Geometry check sheet. Reference: the model listing, model coordinates, mm. Face numbers are marked on the shaded views. A direction names the side the tool comes from. Coordinates: 2 decimals unless noted, no trailing zeros. Write each loop counter-clockwise with the first axis right and the second up, starting at its lowest first coordinate (ties: lowest second). Pieces come first, ordered by that corner, then holes. Notation, with made-up numbers: (62, 45) -> (90, 45) arc R19 cw to (90, 74) -> close; hole circle Ø5 at (37, 17). An arc over 180 degrees is marked (long way). Use a Markdown table: item, result.
Autodesk Inventor part; units mm, degrees
ref_plane "Work Plane1" through (29, 0, 0) normal (0, -1, 0) x (1, 0, 0)
ref_plane "YZ Plane" through (0, 0, 0) normal (1, 0, 0) x (0, 1, 0)
ref_plane "XZ Plane" through (0, 0, 0) normal (0, 1, 0) x (-1, 0, 0)
sketch "Sketch1" plane through (0, 0, 0) normal (0, 0, 1) x (1, 0, 0)
  line L0 (0.1133, 0) -> (20, 0)
  line L1 (20, 0) -> (20, 3)
  line L2 (20, 3) -> (3, 3)
  line L3 (3, 3) -> (2.3864, 3)
  line L4 (2.3864, 3) -> (0, 3)
  line L5 (0, 3) -> (0, 5.25)
  line L6 (0, 5.25) -> (-3.3, 5.25)
  line L7 (-3.3, 5.25) -> (-3.3, 2.3094)
  line L8 (-3.3, 2.3094) -> (-1.22, 2.3094)
  line L9 (-1.22, 2.3094) -> (0.1133, 0)
  line L10 (-7.96, 0) -> (24.66, 0)
  line L11 (0, -1.05) -> (0, 6.3)
  line L12 (3, 3) -> (0, 3) construction
  dimension "d1" = 17
  dimension "d2" = 0.6136
  dimension "d3" = 3.3
  dimension "d4" = 2.08
  dimension "d5" = 60
  dimension "d6" = 6
  dimension "d7" = 6
  dimension "d8" = 4.6188
  dimension "d9" = 10.5
  dimension "d26" = 20
revolve "Body" add sketch "Sketch1" angle 360 about axis through (0.1133, 0, 0) along (1, 0, 0) contours L9 L11 L4 L3 L2 L1 L0 | L9 L8 L7 L6 L5 L11
sketch "Sketch2" plane through (-3.3, 0, 0) normal (-1, 0, 0) x (0, 0, 1)
  circle A0 centre (0, 0) radius 2.3094
  line L0 (0, -7.35) -> (0, 7.35)
  line L1 (-7.35, 0) -> (7.35, 0)
  line L2 (2.3094, 0) -> (1.1547, -2)
  line L3 (1.1547, -2) -> (-1.1547, -2)
  line L4 (-1.1547, -2) -> (-2.3094, 0)
  line L5 (-2.3094, 0) -> (-1.1547, 2)
  line L6 (-1.1547, 2) -> (1.1547, 2)
  line L7 (1.1547, 2) -> (2.3094, 0)
extrude "Slot" add sketch "Sketch2" against normal up to next contours L7 A0 | A0 L2 | L6 L0 A0 | A0 L0 L3 | L0 L6 A0 | A0 L3 L0 | L4 A0 | A0 L5
fillet "Fillet1" radius 2.56 1 edges at (-3.3, -5.25, 0)
thread "Thread"
chamfer "Chamfer1" distance 0.6135 distance2 0.6135 1 edges at (20, -3, 0) measured on face at (20, 1.0659, 1.0214)
ref_plane "Work Plane1" through (29, 0, 0) normal (0, -1, 0) x (1, 0, 0)
fillet "Fillet2" radius 0.5 1 edges at (0, -3, 0)
equation "\"d1\" = GEL"
equation "\"d3\" = KOH"
equation "\"d4\" = INTI"
equation "\"d6\" = GD"
equation "\"d7\" = BDM"
equation "\"d8\" = 1.1547 * SW"
equation "\"d9\" = KOD"
equation "\"d26\" = NLG"
equation "\"d30\" = R"
equation "\"d17\" = RR"
equation "\"d13\" = GEL"
equation "\"d15\" = -0.5 * SPD + 0.5 * GD"
equation "\"d16\" = GUL"
equation "\"GD\" = NND"
equation "\"NLG\" = 20"
equation "\"GEL\" = 17"
equation "\"KOD\" = 10.5"
equation "\"KOH\" = 3.3"
equation "\"INTI\" = 2.08"
equation "\"GAL\" = 0.61345 * PTC"
equation "\"GUL\" = 0.61345 * PTC"
equation "\"BDM\" = NND"
equation "\"SW\" = 4"
equation "\"RR\" = 2.56"
equation "\"SPD\" = NND - 1.2269 * PTC"
equation "\"R\" = 0.5"
equation "\"TOA\" = 30deg"
equation "\"GD1\" = THREADDIA - 1.2269 * PTC"
equation "\"THREADDIA\" = 6"
equation "\"PTC\" = 1"
equation "\"NND\" = 6"
equation "\"KOH1\" = 0.74"
equation "\"E0\" = 4.583"
properties part number "ISO 7380-1 - M6 x 20" material "Steel"
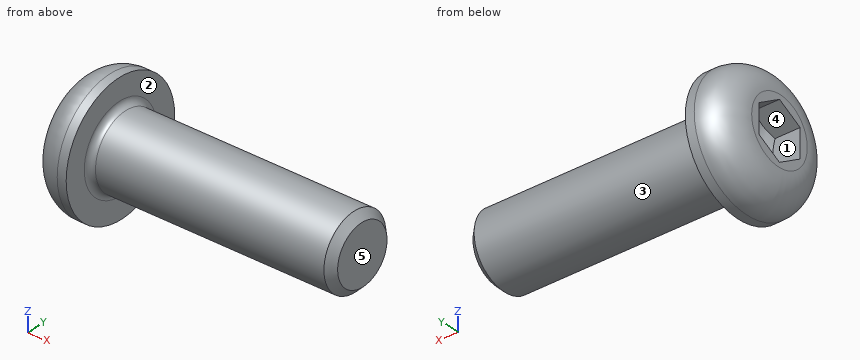
Item 1: Mould release check, pull along Y, two halves, no side actions. Record for the marked faces 3, 4 and 5: +Y half, -Y half, draft (parallel to the pull), parting line (faces both ways), or undercut.
Answer block:
| item | result |
|---|---|
| face 3 | parting line |
| face 4 | undercut |
| face 5 | draft |
Item 2: Depth check by flat-ended pin: P1, Ø1.5, axis at x = 2.5, y = -3, coming from the -Z side; P2, Ø2, axis at x = 12, y = -3.5, coming from the -Z side; P3, Ø4, axis at x = 6, z = -0.5, coming from the +Y side. Enter the tip coordinate at first touch or a pass-through.
Answer block:
| item | result |
|---|---|
| P1 | stops at z = -1.98 |
| P2 | stops at z = -1.66 |
| P3 | stops at y = 3 |
Item 3: Tool access check on the marked faces 1 and 2. Record the directions out of +Z, -Z, +X, -X, +Y, -Y that give a thin tool (end or side, any length) a straight path to the whole face; none if there is none.
Answer block:
| item | result |
|---|---|
| face 1 | -X |
| face 2 | +X |
Item 4: Thickness scan on L1, parallel to X at y = 0, z = -4.25; L2, parallel to Y at x = 13.75, z = -0.25; L3, parallel to Z at x = 14, y = 2. Record the ranges inside material, lowest first. Write a range as [from, to].
Answer block:
| item | result |
|---|---|
| L1 | x = [-2.77, 0] |
| L2 | y = [-2.99, 2.99] |
| L3 | z = [-2.24, 2.24] |
Item 5: Section check A-A on x = 12. Record the boundary of the cut face in (y, z).
Answer block:
| item | result |
|---|---|
| outline | circle Ø6 at (0, 0) |
